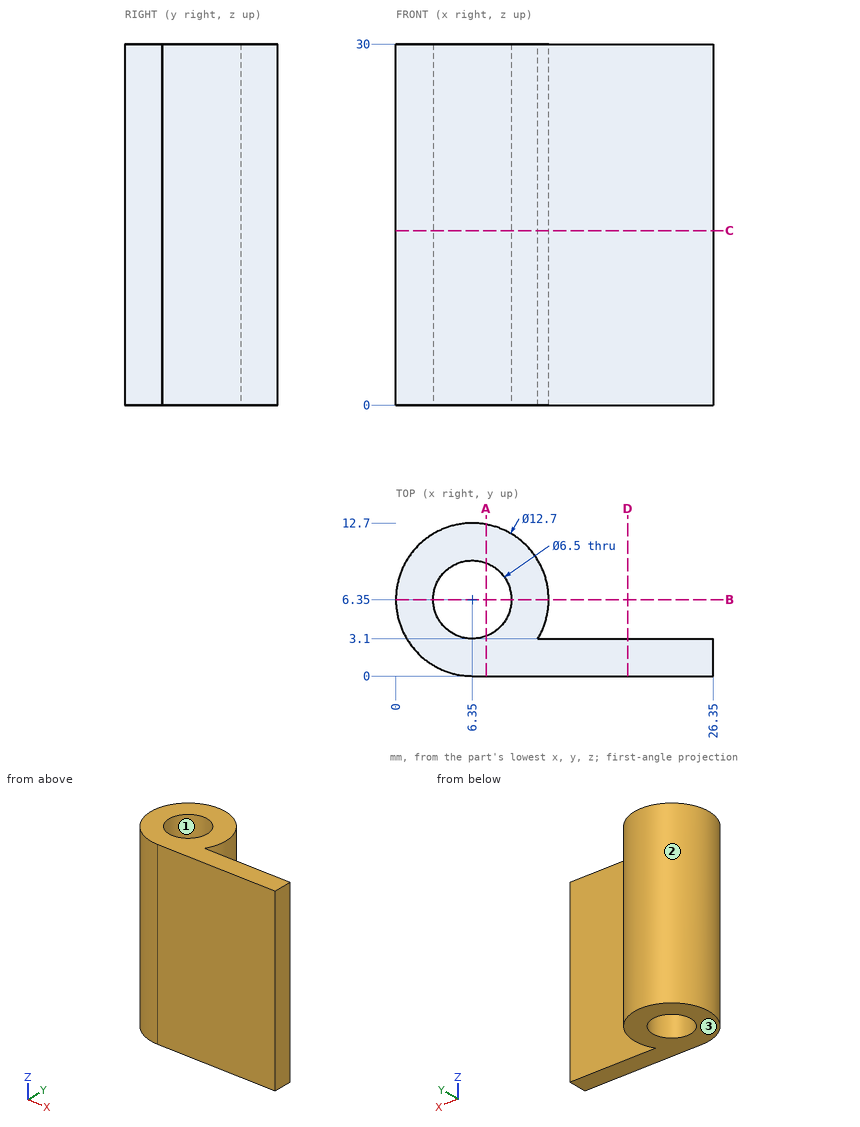
Could you check a few things on this drawing? It's one solid part, dimensions in mm from its lowest x, y, z. Round coordinates to 2 decimals unless told otherwise and drop trailing zeros. Order: outer loops, then holes, each group sorted by start corner. A loop starts at its lowest first (then second) coordinate and runs counter-clockwise, first axis right, second up. Notation, with made-up numbers: (38, 41) -> (45, 41) arc R29 ccw to (45, 74) -> close; hole circle Ø7 at (47, 18.5). An arc over 180 degrees is marked (long way). One line per question, with ' | ' between items.
Q1. If we section it at B-B on y = 6.35: Write out the boundary of the cut face in (x, z), plus the area to 3 significant figures.
Computed values:
outline: (0, 0) -> (3.1, 0) -> (3.1, 30) -> (0, 30) -> close; (9.6, 0) -> (12.7, 0) -> (12.7, 30) -> (9.6, 30) -> close | area: 186 mm²
Q2. If we section it at D-D on x = 19.25: Write out the boundary of the cut face in (y, z), plus the area to 3 significant figures.
Computed values:
outline: (0, 0) -> (3.1, 0) -> (3.1, 30) -> (0, 30) -> close | area: 93.0 mm²
Q3. We'd pull the mould along X, two halves only. Please class the marked faces 1, 2 and 3: released by +X, released by -X, zero draft, split by the parting line, or undercut.
Computed values:
face 1: undercut | face 2: split by the parting line | face 3: zero draft
Q4. I'm going to push flat-ended pins straight in: pin 1 (5 mm diameter, centred on y = 10.5, z = 6, fed in from +X); pin 2 (7.5 mm diameter, centred on x = 6.35, y = 6.35, fed in from +Z); pin 3 (7.5 mm diameter, centred on x = 20, z = 11.5, fed in from +Y); pin 4 (3 mm diameter, centred on x = 14.5, y = 5, fed in from +Z). Where does each tip first touch, or does it pass through?
Computed values:
pin 1: x = 12.48 | pin 2: z = 30 | pin 3: y = 3.1 | pin 4: through
Q5. If I drill on line 1 (Y direction, x = 6.35, z = 17.75); line 2 (X direction, y = 4.75, z = 5.75), over which ranges is the centre line in solid material (lowest first)? Write a range as from..to.
Computed values:
line 1: 0..3.1, 9.6..12.7 | line 2: 0.2..3.52, 9.18..12.5
Q6. If we section it at A-A on x = 7.5: Write out the boundary of the cut face in (y, z) (3 decimals), plus the area to 3 significant figures.
Computed values:
outline: (0, 0) -> (3.31, 0) -> (3.31, 30) -> (0, 30) -> close; (9.39, 0) -> (12.595, 0) -> (12.595, 30) -> (9.39, 30) -> close | area: 195 mm²
Q7. If we section it at C-C on z = 14.5: Write out the boundary of the cut face in (x, y), plus the area to 3 significant figures.
Computed values:
outline: (6.35, 0) -> (26.35, 0) -> (26.35, 3.1) -> (11.81, 3.1) arc R6.35 ccw (long way) to start; hole circle Ø6.5 at (6.35, 6.35) | area: 144 mm²
